Here's the drawing with two shaded views (mm, measured from the low corner). I have some questions. A direction names the side the tool comes from. Round coordinates to 2 decimals unless told otherwise and drop trailing zeros. Loops run counter-clockwise (first coordinate to the right, second up) from the corner with the lowest first, then second, coordinate; pieces in that order, holes last. Notation, with made-up numbers: (-39, 0) - (8, 0) arc R18 ccw to (8, 23) - close; hole circle Ø5 at (39, 15). An arc over 180 degrees is marked (long way). Use one line per item in the form item = value.
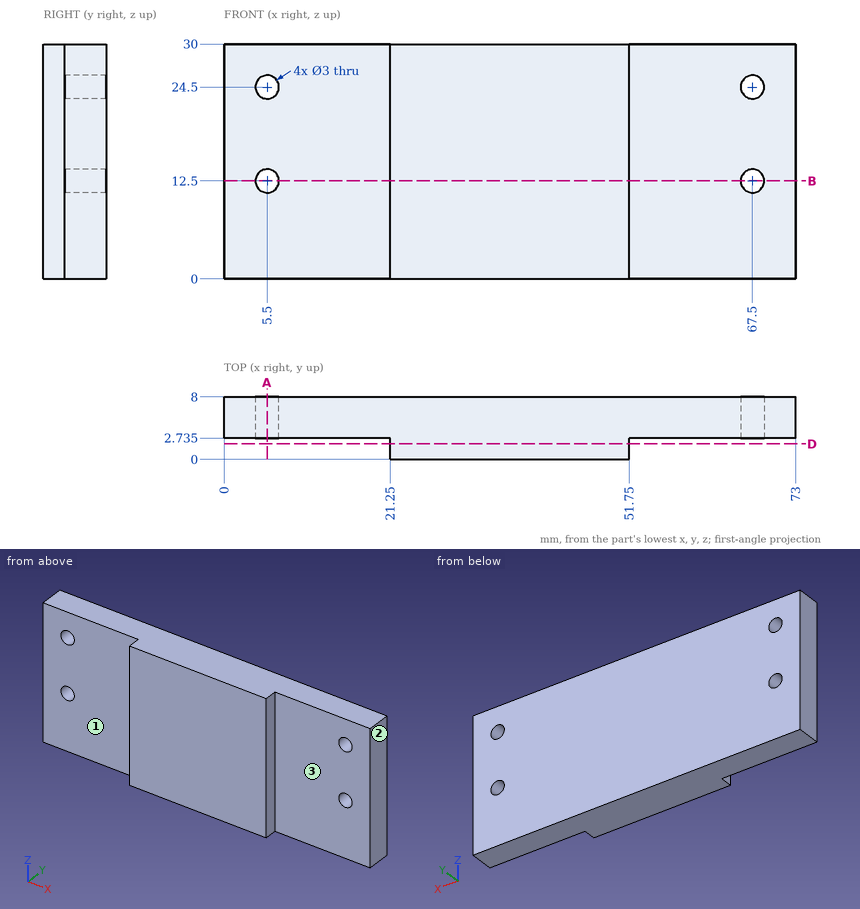
1. If we section it at A-A, the plane x = 5.5: Write out the boundary of the cut face in (y, z) (1 decimal).
Solution:
outline = (2.7, 0) - (8, 0) - (8, 11) - (2.7, 11) - close; (2.7, 14) - (8, 14) - (8, 23) - (2.7, 23) - close; (2.7, 26) - (8, 26) - (8, 30) - (2.7, 30) - close
2. For P1, Ø1.5, axis at y = 1.5, z = 17, coming from the -X side; P2, Ø10.5, axis at x = 13.5, z = 8, coming from the -Y side (1 decimal), each with a flat end and sliding along its axis, tell me the tip position at first contact or that it passes through.
Solution:
P1 = 21.25
P2 = 2.7
3. On a 3-axis mill with a long thin cutter (end or side, diameter ignored), from which of +Z, -Z, +X, -X, +Y, -Y can I reach the whole of each face in a straight line? I mean the marked faces 1, 2 and 3. Say none if no direction works.
Solution:
face_1 = +Z, -Z, -X, -Y
face_2 = +Z, -Z, +X, +Y, -Y
face_3 = +Z, -Z, +X, -Y
4. Please list where these lines run through material, in increasing order: line 1 along Z through (x, y) = (67.5, 6.15); line 2 along Y through (x, z) = (20.5, 21) (1 decimal); line 3 along X through (y, z) = (3, 11.5).
Solution:
line_1 = 0 to 11, 14 to 23, 26 to 30
line_2 = 2.7 to 8
line_3 = 0 to 4.38, 6.62 to 66.38, 68.62 to 73
5. If we section it at D-D, the plane y = 2: Write out the boundary of the cut face in (x, z).
Solution:
outline = (21.25, 0) - (51.75, 0) - (51.75, 30) - (21.25, 30) - close
6. If we section it at B-B, the plane z = 12.5: Count the separate pieces of the cut face and the enclosed holes in it, plus the area to 3 significant figures.
Solution:
separate_pieces = 3
enclosed_holes = 0
area = 436 mm^2
